```python
from build123d import *

# Parameters (mm, degrees)
F0_R           = 11.15
F1_DEPTH       = 52
F2_D           = 3
F2_CSINK_D     = 5
F2_CSINK_ANGLE = 90
F3_W           = 44.3
F3_H           = 47
F4_DEPTH       = 45
F5_SIZE        = 45


with BuildPart() as f1:
    # F0 (on Top) → F1 (new body)
    with BuildSketch(Plane.XY):
        with BuildLine():
            Line((60, -4.2347954512), (60, 30.7652045488))
            Line((60, 30.7652045488), (-60, 30.7652045488))
            Line((-60, 30.7652045488), (-60, -21.2347954512))
            Line((-60, -21.2347954512), (-13.7, -21.2347954512))
            Line((-13.7, -21.2347954512), (-13.7, -4.2347954512))
            Line((-13.7, -4.2347954512), (-7.7, -4.2347954512))
            ThreePointArc((-7.7, -4.2347954512), (20, 23.4652045488), (47.7, -4.2347954512))
            Line((47.7, -4.2347954512), (60, -4.2347954512))
        make_face()
        with Locations((-36, 0.7652045488)):
            Circle(F0_R, mode=Mode.SUBTRACT)
    extrude(amount=-F1_DEPTH)

    # F2 (through all)
    with Locations(Plane.XY):
        with Locations((-51.5, 16.2652045488), (-20.5, 16.2652045488), (-51.5, -14.7347954512), (-20.5, -14.7347954512)):
            CounterSinkHole(F2_D / 2, F2_CSINK_D / 2, counter_sink_angle=F2_CSINK_ANGLE)

    # F3 (on face) → F4 (cut)
    with BuildSketch(Plane.XZ.offset(21.2347954512)):
        with Locations((-35.85, -28.5)):
            Rectangle(F3_W, F3_H)
    extrude(amount=-F4_DEPTH, mode=Mode.SUBTRACT)

    # F5
    f5_edges = [f1.edges().sort_by_distance(p)[0] for p in [
        (-59, -21.234795, -52),
    ]]
    chamfer(f5_edges, length=F5_SIZE)


solid = f1.part
```
Check sheet for the modelled part. Datum: model origin and axes. Units: mm. A direction names the side the tool comes from. Round coordinates to 2 decimals unless told otherwise and drop trailing zeros. Loops run counter-clockwise (first coordinate to the right, second up) from the corner with the lowest first, then second, coordinate; pieces in that order, holes last. Notation, with made-up numbers: (9.25, -25.5) - (21.25, -25.5) arc R28 ccw to (21.25, 5.5) - close; hole circle Ø7 at (-20.5, 11). An arc over 180 degrees is marked (long way). Answer as a JSON object with one key per item and string values. Group by question number.
Q1. Scan lines: line 1 along Y through (x, z) = (-20.5, -2.15); line 2 along X through (y, z) = (-2, -18.5); line 3 along X through (y, z) = (10, -3). Record each from-to range of solid material in increasing order. Write a range as [from, to].
Q2. Set-up check for faces 4 (the face through (-11, -4.235, -26)), 5 (the face through (-58, 6, -18)), 6 (the face through (-59.014, 0.95, -29.185)), 7 (the face through (19.39, 23.46, -25.64)), 8 (the face through (-50.394, 17.279, -3.028)): record each of +Z, -Z, +X, -X, +Y, -Y from which the full face is reachable in a straight line by a thin tool's end or side.
Q3. Mould release check, pull along X, two halves, no side actions. Record for faces 1 (the face through (-60, 11, -20)), 2 (the face through (-13.7, -13, -2)), 3 (the face through (-19.394, 17.279, -3.028)): released by +X, released by -X, zero draft, split by the parting line, or undercut.
Q4. Sectioned sample at D-D, the plane z = -15. Enter the section's corners in (x, y).
Q5. Sectioned sample at A-A, the plane x = -36. Enter the section's corners in (y, z), plus the area to 4 significant figures.
Q6. Sectioned sample at B-B, the plane y = 9. Enter the section's corners in (x, z).
Q7. Gauge pin test, flat ends, axial feed: P1, Ø4, axis at x = -33, y = 9, coming from the -Z side; P2, Ø1, axis at x = -31.5, z = -15, coming from the -Y side; P3, Ø4, axis at x = -51.5, y = 16.27, coming from the -Z side; P4, Ø5, axis at y = 0.5, z = -33.5, coming from the -X side. Record the tip position at first contact, or that the pin passes through.
Q8. Sectioned sample at C-C, the plane x = -20.5. Enter the section's corners in (y, z).
Solution:
{
 "1": {"line 1": "y = [-21.23, -16.23], [-13.23, 14.77], [17.77, 30.77]", "line 2": "x = [-60, -58], [-13.7, -7.61], [47.61, 60]", "line 3": "x = [-60, -42.25], [-29.75, -3.76], [43.76, 60]"},
 "2": {"face 4": "+Z, -Z, +X, -Y", "face 5": "-Z, -Y", "face 6": "-Z, -X, -Y", "face 7": "+Z, -Z, -Y", "face 8": "+Z, -Z"},
 "3": {"face 1": "released by -X", "face 2": "released by +X", "face 3": "undercut"},
 "4": {"outline": "(-60, -13.23) - (-58, -13.23) - (-58, 23.77) - (-13.7, 23.77) - (-13.7, -4.23) - (-7.7, -4.23) arc R27.7 cw to (47.7, -4.23) - (60, -4.23) - (60, 30.77) - (-60, 30.77) - close"},
 "5": {"outline": "(-21.23, -5) - (-10.38, -5) - (-10.38, 0) - (-21.23, 0) - close; (11.92, -5) - (23.77, -5) - (23.77, -52) - (30.77, -52) - (30.77, 0) - (11.92, 0) - close", "area": "477.5 mm²"},
 "6": {"outline": "(-60, -37.23) - (-58, -37.23) - (-58, -5) - (-43.52, -5) - (-43.52, 0) - (-60, 0) - close; (-28.48, -5) - (-13.7, -5) - (-13.7, -52) - (-4.33, -52) - (-4.33, 0) - (-28.48, 0) - close; (44.33, -52) - (60, -52) - (60, 0) - (44.33, 0) - close"},
 "7": {"P1": "passes through", "P2": "stops at y = 23.77", "P3": "stops at z = -5", "P4": "stops at x = -13.7"},
 "8": {"outline": "(-21.23, -5) - (-16.23, -5) - (-16.23, -1) - (-17.23, 0) - (-21.23, 0) - close; (-13.23, -5) - (14.77, -5) - (14.77, -1) - (13.77, 0) - (-12.23, 0) - (-13.23, -1) - close; (17.77, -5) - (23.77, -5) - (23.77, -52) - (30.77, -52) - (30.77, 0) - (18.77, 0) - (17.77, -1) - close"}
}
